Read the model definition and answer for the solid it produces. Units are mm, in the model's axes. A direction names the side the tool comes from. Give positions to 0.01 mm unless a question says otherwise; leave off trailing zeros. Loops run counter-clockwise (first coordinate to the right, second up) from the corner with the lowest first, then second, coordinate; pieces in that order, holes last. Notation, with made-up numbers: (-28, -25.5) - (21, -25.5) arc R29 cw to (21, 3.5) - close; hole circle Ø5 at (74, -31.5). An arc over 180 degrees is marked (long way). Write each question's results on one line, items separated by ' | '. Start each with the question number.
Q1. The part is cut by section B-B, the plane z = 2.75. Write down the section's boundary in (x, y), plus the area to 4 significant figures.
Q2. Determine the mould class of faces 5 (the flat face through (10, -2.5, 5)), 6 (the flat face through (20, 4.5, 5)), 7 (the flat face through (-7.5, 0, 5)) for opening direction X: +X half, -X half, draft (parallel to the pull), parting line (faces both ways), or undercut.
Q3. The part is cut by section A-A, the plane y = -3.75. Write down the section's boundary in (x, z).
Q4. For faces 1 (the flat face through (0, -10, 5)), 2 (the flat face through (10, 2.5, 5)), 3 (the flat face through (7.5, -6, 5)), 4 (the flat face through (20, -4.5, 5)), determine the directions among +Z, -Z, +X, -X, +Y, -Y from which every point of the face is accessible in a straight line to the end or side of a thin tool.
Q5. The part is cut by section D-D, the plane y = 8.75. Write down the section's boundary in (x, z), plus the area to 3 significant figures.
Q6. Find the intervals of material crossed by line 1 (X direction, y = 3, z = 5.75); line 2 (X direction, y = 9, z = 2.75); line 3 (Y direction, x = 22.5, z = 2), in increasing order. Write a range as from..to.
Q7. Given pin 1 (1.5 mm diameter, centred on x = 9.5, z = 9, fed in from -Y); pin 2 (2 mm diameter, centred on y = -7, z = 4.5, fed in from +X); pin 3 (2 mm diameter, centred on x = 15.5, z = 2.5, fed in from +Y), each flat-ended and moving along its own axis, determine where each tip first touches the part or whether it passes through.
Q8. The part is cut by section C-C, the plane x = 19.5. Write down the section's boundary in (y, z), plus the area to 3 significant figures.
```python
from build123d import *

# Parameters (mm, degrees)
SKETCH1_W           = 15
SKETCH1_H           = 20
SKETCH1_W_2         = 6
SKETCH1_H_2         = 5
BOSS_EXTRUDE1_DEPTH = 10


with BuildPart() as part:
    # Sketch1 → Boss-Extrude1 (new body)
    with BuildSketch(Plane.XY):
        Rectangle(SKETCH1_W, SKETCH1_H)
        with Locations((10.5, 0)):
            Rectangle(SKETCH1_W_2, SKETCH1_H_2)
        Polygon((13.5, 2.5), (13.5, -2.5), (13.5, -4.5), (26, -4.5), (26, 4.5), (13.5, 4.5), align=None)
    extrude(amount=BOSS_EXTRUDE1_DEPTH)


solid = part.part
```
Check sheet entries:
1) outline: (-7.5, -10) - (7.5, -10) - (7.5, -2.5) - (13.5, -2.5) - (13.5, -4.5) - (26, -4.5) - (26, 4.5) - (13.5, 4.5) - (13.5, 2.5) - (7.5, 2.5) - (7.5, 10) - (-7.5, 10) - close | area: 442.5 mm^2
2) face 5: undercut | face 6: draft | face 7: -X half
3) outline: (-7.5, 0) - (7.5, 0) - (7.5, 10) - (-7.5, 10) - close; (13.5, 0) - (26, 0) - (26, 10) - (13.5, 10) - close
4) face 1: +Z, -Z, +X, -X, -Y | face 2: +Z, -Z, +Y | face 3: +Z, -Z, -Y | face 4: +Z, -Z, +X, -Y
5) outline: (-7.5, 0) - (7.5, 0) - (7.5, 10) - (-7.5, 10) - close | area: 150 mm^2
6) line 1: x = -7.5..7.5, 13.5..26 | line 2: x = -7.5..7.5 | line 3: y = -4.5..4.5
7) pin 1: stops at y = -2.5 | pin 2: stops at x = 7.5 | pin 3: stops at y = 4.5
8) outline: (-4.5, 0) - (4.5, 0) - (4.5, 10) - (-4.5, 10) - close | area: 90.0 mm^2
